Autodesk Inventor part; units mm, degrees
ref_plane "YZ Plane" through (0, 0, 0) normal (1, 0, 0) x (0, 1, 0)
ref_plane "XZ Plane" through (0, 0, 0) normal (0, 1, 0) x (-1, 0, 0)
ref_plane "XY Plane" through (0, 0, 0) normal (0, 0, 1) x (1, 0, 0)
sketch "Sketch1" plane through (0, 0, 0) normal (0, 0, 1) x (1, 0, 0)
  line L0 (-20, -20) -> (20, -20)
  line L1 (20, -20) -> (20, 20)
  line L2 (20, 20) -> (-20, 20)
  line L3 (-20, 20) -> (-20, -20)
  line L4 (-20, -20) -> (20, 20) construction
  line L5 (20, -20) -> (-20, 20) construction
  line L6 (-5, -3) -> (5, -3)
  line L7 (5, -3) -> (5, 3)
  line L8 (5, 3) -> (-5, 3)
  line L9 (-5, 3) -> (-5, -3)
  line L10 (-5, -3) -> (5, 3) construction
  line L11 (5, -3) -> (-5, 3) construction
  point P0 (0, 0)
  dimension "d2" = 40
  dimension "d3" = 40
  dimension "d6" = 10
  dimension "d7" = 6
extrude "Extrusion1" add sketch "Sketch1" along normal blind 6 contours L3 L2 L1 L0 | L9 L8 L7 L6
extrude "Extrusion2" cut sketch "Sketch1" along normal through all contours L9 L8 L7 L6
properties part number "Push_1"
Geometry: final body of the model. Coordinates: model frame, mm. A direction names the side the tool comes from. Give positions to 0.01 mm unless a question says otherwise; leave off trailing zeros. Order: outer loops, then holes, each group sorted by start corner. A loop starts at its lowest first (then second) coordinate and runs counter-clockwise, first axis right, second up. Notation, with made-up numbers: (58, 51.25) -> (95, 51.25) arc R20 cw to (95, 71.25) -> close; hole circle Ø8 at (54.5, 86). An arc over 180 degrees is marked (long way). Write each question's results on one line, items separated by ' | '. Start each with the question number.
1) Set-up query: faces 1 (the flat face through (0, -3, 3)), 2 (the flat face through (0, -20, 3)). Return all of +Z, -Z, +X, -X, +Y, -Y with unobstructed straight access to the full face (end or side cutting, diameter ignored); none if empty.
2) Draft query along X for faces 3 (the flat face through (-20, 0, 3)), 4 (the flat face through (0, 5, 0)), 5 (the flat face through (5, 0, 3)). Return one class per face: pulls with the +X half, pulls with the -X half, needs draft (parallel to the pull), parting line crosses it, or undercut.
3) Section A-A (x = 4). Return loops of the section in (y, z).
4) Line query: line 1 (Y direction, x = 3.5, z = 2.5); line 2 (X direction, y = 2, z = 3.2). Output: solid intervals per line, ascending. Write a range as from..to.
5) Section B-B (y = 1). Return loops of the section in (x, z).
6) Section C-C (z = 1). Return loops of the section in (x, y), then the cut area to 3 significant figures.
Calculated:
1) face 1: +Z, -Z | face 2: +Z, -Z, +X, -X, -Y
2) face 3: pulls with the -X half | face 4: needs draft | face 5: undercut
3) outline: (-20, 0) -> (-3, 0) -> (-3, 6) -> (-20, 6) -> close; (3, 0) -> (20, 0) -> (20, 6) -> (3, 6) -> close
4) line 1: -20..-3, 3..20 | line 2: -20..-5, 5..20
5) outline: (-20, 0) -> (-5, 0) -> (-5, 6) -> (-20, 6) -> close; (5, 0) -> (20, 0) -> (20, 6) -> (5, 6) -> close
6) outline: (-20, -20) -> (20, -20) -> (20, 20) -> (-20, 20) -> close; hole (-5, -3) -> (5, -3) -> (5, 3) -> (-5, 3) -> close | area: 1,540 mm2
